from build123d import *

# Parameters (mm, degrees)
SKETCH003_W = 8.5
SKETCH003_H = 3
FILLET_R    = 1


with BuildPart() as part:
    # Sketch003 → Revolution002 (revolve)
    with BuildSketch(Plane.XZ):
        with Locations((4.25, 35.166221)):
            Rectangle(SKETCH003_W, SKETCH003_H)
    revolve(axis=Axis((0, 0, 0), (0, 0, 1)))

    # Fillet
    fillet_edges = [part.edges().sort_by_distance(p)[0] for p in [
        (-8.5, 0, 36.666221),
    ]]
    fillet(fillet_edges, radius=FILLET_R)

    # Sketch004 → Groove (revolve, cut)
    with BuildSketch(Plane.XZ):
        Polygon((0, 36.666221), (0, 29.34667), (1.5, 29.34667), (1.5, 34.966221), (3.2, 36.666221), align=None)
    revolve(axis=Axis((0, 0, 0), (0, 0, 1)), mode=Mode.SUBTRACT)


solid = part.part
Part model, mm, in its own coordinate system. Coordinates: 2 decimals unless noted, no trailing zeros. Loops run counter-clockwise (first coordinate to the right, second up) from the corner with the lowest first, then second, coordinate; pieces in that order, holes last. Notation, with made-up numbers: (-37, -33.75) - (-19, -33.75) arc R20 cw to (-19, -11.75) - close; hole circle Ø9 at (71.5, 62.25). An arc over 180 degrees is marked (long way). Write each question's results on one line, items separated by ' | '. Start each with the question number.
Q1. Slice it at A-A on x = 0. Give the cut face in (y, z), and give its area (3 significant figures).
Q2. Probe line 1 along Y through (x, z) = (0, 34.05); line 2 along X through (y, z) = (-2.5, 36.4); line 3 along Y through (x, z) = (-4, 35.05). List the from-to ranges inside material, lowest first.
Q3. Slice it at D-D on z = 36.05. Give the cut face in (x, y).
Q4. Drop a flat-ended pin along its axis: pin 1 Ø1 at (y, z) = (-2.5, 35) entering from +X. Give the stop position or say it passes through.
Q5. Slice it at C-C on z = 34.2. Give the cut face in (x, y), and give its area (3 significant figures).
Q6. Two-plate mould, pull along Y, no slides. Class faces 1 (the cylindrical face through (-1.5, 0.07, 34.33)), 2 (the cylindrical face through (4.57, 7.167, 34.68)), 3 (the flat face through (-2, 0, 33.666)): +Y half, -Y half, draft (parallel to the pull), parting line (faces both ways), or undercut.
Answer:
1) outline: (-8.5, 33.67) - (-1.5, 33.67) - (-1.5, 34.97) - (-3.2, 36.67) - (-7.5, 36.67) arc R1 ccw to (-8.5, 35.67) - close; (1.5, 33.67) - (8.5, 33.67) - (8.5, 35.67) arc R1 ccw to (7.5, 36.67) - (3.2, 36.67) - (1.5, 34.97) - close | area: 38.7 mm2
2) line 1: y = -8.5 to -1.5, 1.5 to 8.5 | line 2: x = -7.79 to -1.54, 1.54 to 7.79 | line 3: y = -7.5 to 7.5
3) outline: circle Ø16.85 at (0, 0); hole circle Ø5.17 at (0, 0)
4) pin 1: stops at x = 8.26
5) outline: circle Ø17 at (0, 0); hole circle Ø3 at (0, 0) | area: 220 mm2
6) face 1: undercut | face 2: parting line | face 3: draft
